```python
from build123d import *

# Parameters (mm, degrees)
ESTRUSIONE_ESTRUSIONE1_DEPTH  = 100
TAGLIO_ESTRUSIONE1_DEPTH      = 119.966381806
TAGLIO_ESTRUSIONE1_DEPTH_BACK = 119.966381806
TAGLIO_ESTRUSIONE2_DEPTH      = 142.966381806
TAGLIO_ESTRUSIONE2_DEPTH_BACK = 5
TAGLIO_ESTRUSIONE2_START      = -23
SCHIZZO3_R                    = 19
FORO_20_0_20_1_D              = 20
FORO_10_0_10_1_D              = 10


with BuildPart() as part:
    # Schizzo1 → Estrusione-Estrusione1 (new body)
    with BuildSketch(Plane(origin=(0, 0, 0), x_dir=(0, 0, -1), z_dir=(1, 0, 0))):
        Polygon((0, 48), (0, 0), (-43, 0), (-43, 10), (-20, 10), (-20, 39), (-10, 39), (-10, 48), align=None)
    extrude(amount=ESTRUSIONE_ESTRUSIONE1_DEPTH)

    # Schizzo2 → Taglio-Estrusione1 (cut, two sides: drawn at the far end of the back side and taken through both)
    with BuildSketch(Plane.XY.offset(-TAGLIO_ESTRUSIONE1_DEPTH_BACK)):
        Polygon((-60.289310715, 234.748012024), (70, 48), (100, 5), (230.289310715, -181.748012024), (603.785334763, 78.830609405), (313.206713334, 495.326633453), align=None)
    extrude(amount=TAGLIO_ESTRUSIONE1_DEPTH + TAGLIO_ESTRUSIONE1_DEPTH_BACK, mode=Mode.SUBTRACT)

    # Schizzo3 → Taglio-Estrusione2 (cut, two sides: drawn at the far end of the back side and taken through both)
    with BuildSketch(Plane.XY.offset(43).offset(TAGLIO_ESTRUSIONE2_START - TAGLIO_ESTRUSIONE2_DEPTH_BACK)):
        with Locations((30, 23)):
            Circle(SCHIZZO3_R)
    extrude(amount=TAGLIO_ESTRUSIONE2_DEPTH + TAGLIO_ESTRUSIONE2_DEPTH_BACK, mode=Mode.SUBTRACT)

    # Foro Ø20.0 (20)-1 (through all)
    with Locations(Plane.XY.offset(15)):
        with Locations((30, 23)):
            Hole(FORO_20_0_20_1_D / 2)

    # Foro Ø10.0 (10)-1 (through all)
    with Locations(Plane(origin=(0, 10, 0), x_dir=(1, 0, 0), z_dir=(0, 1, 0))):
        with Locations((80, -32), (60, -32)):
            Hole(FORO_10_0_10_1_D / 2)


solid = part.part
```
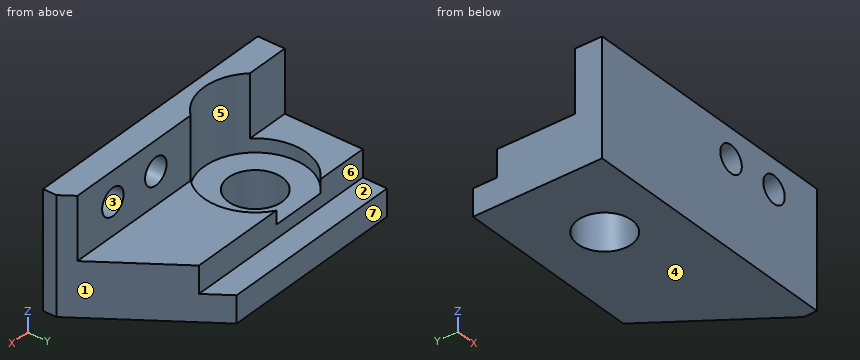
Geometry check sheet. Reference: the model listing, model coordinates, mm. Face numbers are marked on the shaded views. A direction names the side the tool comes from. Give positions to 0.01 mm unless a question says otherwise; leave off trailing zeros. Write each loop counter-clockwise with the first axis right and the second up, starting at its lowest first coordinate (ties: lowest second). Pieces come first, ordered by that corner, then holes.
1) Section check A-A, the plane z = 32. Record the boundary of the cut face in (x, y), and give its area (3 significant figures).
2) Gauge pin test, flat ends, axial feed: pin 1 (8.5 mm diameter, centred on x = 58.5, y = 27, fed in from +Z); pin 2 (5 mm diameter, centred on x = 12, z = 34.5, fed in from +Y); pin 3 (3 mm diameter, centred on y = 14.5, z = 8.5, fed in from +X). Record the tip position at first contact, or that the pin passes through.
3) Access from +Z, -Z, +X, -X, +Y, -Y to the whole of each face (thin tool, end or side, straight path). Record for the marked faces 5, 6 and 7.
4) Section check C-C, the plane z = 3.5. Record the boundary of the cut face in (x, y), and give its area (3 significant figures).
5) Section check D-D, the plane y = 25. Record the boundary of the cut face in (x, z), and give its area (3 significant figures).
6) Material ranges on L1, parallel to X at y = 3, z = 32; L2, parallel to X at y = 8.25, z = 32; L3, parallel to X at y = 8, z = 32, recorded low to high.
7) Section check B-B, the plane x = 60. Record the boundary of the cut face in (y, z), and give its area (3 significant figures).
8) Release check for a two-part mould opening along Z. For the marked faces 1, 2, 3 and 4 record: pulls with the +Z half, pulls with the -Z half, needs draft (parallel to the pull), parting line crosses it, or undercut.
Computed:
1. outline: (0, 0) - (55, 0) - (55, 10) - (43.86, 10) arc R19 cw to (16.14, 10) - (0, 10) - close; (65, 0) - (75, 0) - (75, 10) - (65, 10) - close; (85, 0) - (100, 0) - (100, 5) - (96.51, 10) - (85, 10) - close
1. area: 676 mm2
2. pin 1: stops at z = 20
2. pin 2: stops at y = 10
2. pin 3: stops at x = 94.42
3. face 5: +Z
3. face 6: +Z, +X, -X, +Y
3. face 7: +Z, -Z, +X, -X, +Y
4. outline: (0, 0) - (100, 0) - (100, 5) - (70, 48) - (0, 48) - close; hole circle Ø20 at (30, 23)
4. area: 3,840 mm2
5. outline: (0, 0) - (20.2, 0) - (20.2, 15) - (11.11, 15) - (11.11, 20) - (0, 20) - close; (39.8, 0) - (86.05, 0) - (86.05, 20) - (48.89, 20) - (48.89, 15) - (39.8, 15) - close
5. area: 1,240 mm2
6. L1: x = 0 to 55, 65 to 75, 85 to 100
6. L2: x = 0 to 18.02, 41.98 to 55, 65 to 75, 85 to 97.73
6. L3: x = 0 to 18.34, 41.66 to 55, 65 to 75, 85 to 97.91
7. outline: (0, 0) - (48, 0) - (48, 10) - (39, 10) - (39, 20) - (10, 20) - (10, 27) - (0, 27) - close; (0, 37) - (10, 37) - (10, 43) - (0, 43) - close
7. area: 1,000 mm2
8. face 1: needs draft
8. face 2: pulls with the +Z half
8. face 3: undercut
8. face 4: pulls with the -Z half
